The model under review builds one solid part; all positions refer to its coordinate system, in mm. Give positions to 0.01 mm unless a question says otherwise; leave off trailing zeros. Order: outer loops, then holes, each group sorted by start corner. A loop starts at its lowest first (then second) coordinate and runs counter-clockwise, first axis right, second up.
```python
from build123d import *

# Parameters (mm, degrees)
SKETCH_1_W          = 30
SKETCH_1_H          = 40
EXTRUDE_1_DEPTH     = 3
SKETCH_2_R          = 1.5
CUT_EXTRUDE_1_DEPTH = 10
FILLET_1_R          = 2


with BuildPart() as part:
    # 草图1 → 凸台-拉伸1 (new body)
    with BuildSketch(Plane.XY):
        Rectangle(SKETCH_1_W, SKETCH_1_H)
    extrude(amount=EXTRUDE_1_DEPTH)

    # 草图2 → 切除-拉伸1 (cut)
    with BuildSketch(Plane.XY.offset(3)):
        with Locations((10, 15)):
            Circle(SKETCH_2_R)
        with Locations((-10, 15)):
            Circle(SKETCH_2_R)
        with Locations((10, -15)):
            Circle(SKETCH_2_R)
        with Locations((-10, -15)):
            Circle(SKETCH_2_R)
    extrude(amount=-CUT_EXTRUDE_1_DEPTH, mode=Mode.SUBTRACT)

    # 圆角1
    fillet_1_edges = [part.edges().sort_by_distance(p)[0] for p in [
        (0, -20, 0),
        (-15, 0, 0),
        (0, 20, 0),
        (15, 0, 0),
        (15, -20, 1.5),
        (-15, -20, 1.5),
        (-15, 20, 1.5),
        (15, 20, 1.5),
    ]]
    fillet(fillet_1_edges, radius=FILLET_1_R)


solid = part.part
```
Item 1: Take a section at D-D (y = 10). Give the boundary of the cut face in (x, z), and give its area (3 significant figures).
Values found:
outline: (-15, 2) arc R2 ccw to (-13, 0) - (13, 0) arc R2 ccw to (15, 2) - (15, 3) - (-15, 3) - close
area: 88.3 mm2
Item 2: Take a section at C-C (y = 15). Give the boundary of the cut face in (x, z), and give its area (3 significant figures).
Values found:
outline: (-15, 2) arc R2 ccw to (-13, 0) - (-11.5, 0) - (-11.5, 3) - (-15, 3) - close; (-8.5, 0) - (8.5, 0) - (8.5, 3) - (-8.5, 3) - close; (11.5, 0) - (13, 0) arc R2 ccw to (15, 2) - (15, 3) - (11.5, 3) - close
area: 70.3 mm2
Item 3: Draft analysis for pull direction Y (two halves, no side actions). For faces 1 (the flat face through (-0.2, -20, 2.5)), 2 (the cylindrical face through (8.5, -14.93, 1.52)), 3 (the flat face through (-0.2, 20, 2.5)), state which applies: released by +Y, released by -Y, zero draft, split by the parting line, or undercut.
Values found:
face 1: released by -Y
face 2: undercut
face 3: released by +Y
Item 4: Take a section at B-B (z = 0.8). Give the boundary of the cut face in (x, y), and give its area (3 significant figures).
Values found:
outline: (-14.6, -18) arc R1.6 ccw to (-13, -19.6) - (13, -19.6) arc R1.6 ccw to (14.6, -18) - (14.6, 18) arc R1.6 ccw to (13, 19.6) - (-13, 19.6) arc R1.6 ccw to (-14.6, 18) - close; hole circle Ø3 at (-10, -15); hole circle Ø3 at (-10, 15); hole circle Ø3 at (10, -15); hole circle Ø3 at (10, 15)
area: 1,110 mm2
Item 5: Clearance check with a flat-ended pin moving along its axis: pin 1 Ø2.5 at (x, y) = (10, 15) entering from +Z. State where the tip first meets the part, or that it passes through.
Values found:
pin 1: passes through
Item 6: For line 1 (Y direction, x = 10, z = 1.8); line 2 (Y direction, x = -10, z = 1.1); line 3 (X direction, y = -16, z = 2), list the stretches that pass through material, from the lowest coordinate up.
Values found:
line 1: y = -19.99 to -16.5, -13.5 to 13.5, 16.5 to 19.99
line 2: y = -19.79 to -16.5, -13.5 to 13.5, 16.5 to 19.79
line 3: x = -15 to -11.12, -8.88 to 8.88, 11.12 to 15
Item 7: Take a section at A-A (x = -10). Give the boundary of the cut face in (y, z).
Values found:
outline: (-20, 2) arc R2 ccw to (-18, 0) - (-16.5, 0) - (-16.5, 3) - (-20, 3) - close; (-13.5, 0) - (13.5, 0) - (13.5, 3) - (-13.5, 3) - close; (16.5, 0) - (18, 0) arc R2 ccw to (20, 2) - (20, 3) - (16.5, 3) - close
